```python
from build123d import *


with BuildPart() as part:
    # Sweep1: sweep along a path in Sketch3
    with BuildLine(Plane(origin=(0, 0, 0), x_dir=(1, 0, 0), z_dir=(0, 1, 0))) as sweep1_path:
        Line((12.5, 0), (12.5, 25))
        ThreePointArc((12.5, 25), (8.071891388, 45.571891388), (-4.428108612, 62.5))
        ThreePointArc((-4.428108612, 62.5), (-16.928108612, 79.428108612), (-21.356217223, 100))
        Line((-21.356217223, 100), (-21.356217223, 150))
    # Sketch1 → Sweep1 (sweep)
    with BuildSketch(Plane.XY):
        Polygon((17.394366197, 10), (25, 10), (25, 0), (0, 0), (0, 10), (7.394366197, 10), (7.394366197, 31.044600939), (17.394366197, 31.044600939), align=None)
    sweep(path=sweep1_path.line)


solid = part.part
```
The model under review builds one solid part; all positions refer to its coordinate system, in mm. A direction names the side the tool comes from. Give positions to 0.01 mm unless a question says otherwise; leave off trailing zeros. Write each loop counter-clockwise with the first axis right and the second up, starting at its lowest first coordinate (ties: lowest second). Pieces come first, ordered by that corner, then holes.
(1) Consider section A-A, the plane z = -131. Give the boundary of the cut face in (x, y), and give its area (3 significant figures).
(2) Tool access review of faces 1 (the flat face through (17.394, 20, -13)), 2 (the flat face through (-26.462, 21, -125)), 3 (the flat face through (3, 10, -70)), 4 (the flat face through (0, 5, -13)), 5 (the flat face through (-21, 10, -75)): name each direction out of +Z, -Z, +X, -X, +Y, -Y from which nothing blocks a thin tool from reaching the whole face with its end or side.
(3) Consider section D-D, the plane y = 5.5. Give the boundary of the cut face in (x, z) (3 decimals), and give its area (3 significant figures).
(4) To check wall thickness, follow L1, parallel to X at y = 27, z = -25; L2, parallel to Y at x = 4, z = -25.5; L3, parallel to X at y = 9.5, z = -26. State the ranges of each line that lie inside material, in increasing order.
(5) Consider section B-B, the plane y = 25. Give the boundary of the cut face in (x, z), and give its area (3 significant figures).
(6) For P1, Ø12, axis at y = 4, z = -60, coming from the +X side; P2, Ø17, axis at y = 21.5, z = -11.5, coming from the +X side; P3, Ø6.5, axis at y = 18, z = -115.5, coming from the -X side, all flat-tipped, find the tip position at first contact; note any pin that passes through.
(7) Consider section C-C, the plane x = -14.5. Give the boundary of the cut face in (y, z).
Returned:
1. outline: (-33.86, 0) - (-8.86, 0) - (-8.86, 10) - (-16.46, 10) - (-16.46, 31.04) - (-26.46, 31.04) - (-26.46, 10) - (-33.86, 10) - close
1. area: 460 mm2
2. face 1: +Z, -Z, +X, +Y
2. face 2: +Z, -Z, -X, +Y
2. face 3: -Z, +X, +Y
2. face 4: +Z, -X, +Y, -Y
2. face 5: +Z, -X, +Y
3. outline: (-33.856, -150) - (-8.856, -150) - (-8.856, -100) arc R37.5 cw to (3.84, -71.875) arc R62.5 ccw to (25, -25) - (25, 0) - (0, 0) - (0, -25) arc R37.5 cw to (-12.696, -53.125) arc R62.5 ccw to (-33.856, -100) - close
3. area: 4,000 mm2
4. L1: x = 7.39 to 17.39
4. L2: y = 0 to 10
4. L3: x = -0.01 to 24.99
5. outline: (-26.46, -150) - (-16.46, -150) - (-16.46, -100) arc R45.11 cw to (-1.19, -66.17) arc R54.89 ccw to (17.39, -25) - (17.39, 0) - (7.39, 0) - (7.39, -25) arc R44.89 cw to (-7.81, -58.67) arc R55.11 ccw to (-26.46, -100) - close
5. area: 1,600 mm2
6. P1: stops at x = 17.86
6. P2: stops at x = 17.39
6. P3: stops at x = -26.46
7. outline: (0, -150) - (10, -150) - (10, -86.84) - (31.04, -86.84) - (31.04, -65.72) - (10, -65.72) - (10, -54.78) - (0, -54.78) - close
